Model file for the job. Use its own axes, mm. Give positions to 0.01 mm unless a question says otherwise; leave off trailing zeros. Write each loop counter-clockwise with the first axis right and the second up, starting at its lowest first coordinate (ties: lowest second). Pieces come first, ordered by that corner, then holes. Notation, with made-up numbers: M 71,52 L 89,52 A14 ccw 89,75 Z; hole C 6.25,50 d1. An arc over 180 degrees is marked long. Answer as a JSON object with one key per item and string values. Group by question number.
Solid Edge part; units mm, degrees
sketch "Sketch1" plane through (0, 0, 0) normal (0, -1, 0) x (1, 0, 0)
  circle A0 centre (0, 0) radius 6.1
extrude "Protrusion1" add sketch "Sketch1" along normal mid plane 19
chamfer "Chanfro_1" distance 1.5 angle 45 1 edges at (-6.1, 9.5, 0) measured on face at (-3.9447, 9.5, 4.1887)
chamfer "Chanfro_2" distance 1.5 angle 45 1 edges at (-6.1, -9.5, 0) measured on face at (-3.9447, -9.5, 4.1887)
Q1. Drop flat-ended pins along their axis: P1, Ø1, axis at y = 5, z = 2.5, coming from the -X side; P2, Ø2, axis at x = -4.5, z = 4.5, coming from the -Y side. Give the stop position or say it passes through.
Q2. Slice it at C-C, the plane y = 0.25. Write the cut outline in (x, z), then the cut area to 3 significant figures.
Q3. Wall check: L1, parallel to X at y = -5, z = 4; L2, parallel to Y at x = 3.75, z = -4.75; L3, parallel to X at y = 0, z = -3.75. Give the ranges that are in metal, low to high.
Q4. Slice it at A-A, the plane z = 0. Write the cut outline in (x, y), then the cut area to 3 significant figures.
Q5. Slice it at B-B, the plane x = 0. Write the cut outline in (y, z).
Solved:
{
 "1": {"P1": "stops at x = -5.76", "P2": "stops at y = -8.74"},
 "2": {"outline": "C 0,0 d12.2", "area": "117 mm²"},
 "3": {"L1": "x = -4.61 to 4.61", "L2": "y = -8.05 to 8.05", "L3": "x = -4.81 to 4.81"},
 "4": {"outline": "M -6.1,-8 L -4.6,-9.5 L 4.6,-9.5 L 6.1,-8 L 6.1,8 L 4.6,9.5 L -4.6,9.5 L -6.1,8 Z", "area": "227 mm²"},
 "5": {"outline": "M -9.5,-4.6 L -8,-6.1 L 8,-6.1 L 9.5,-4.6 L 9.5,4.6 L 8,6.1 L -8,6.1 L -9.5,4.6 Z"}
}
